Here's how the part is built. I have some questions about the finished solid (model axes, mm). A direction names the side the tool comes from. Coordinates: 2 decimals unless noted, no trailing zeros. Loops run counter-clockwise (first coordinate to the right, second up) from the corner with the lowest first, then second, coordinate; pieces in that order, holes last. Notation, with made-up numbers: (-35, -5) -> (-18, -5) arc R32 cw to (-18, 33) -> close; hole circle Ø1 at (4.5, 63). An arc over 180 degrees is marked (long way). Answer as a JSON object with one key per item and string values. Group by question number.
Q1. I want a section at B-B on z = 2.2. Write out the boundary of the cut face in (x, y).
Q2. On a 3-axis mill with a long thin cutter (end or side, diameter ignored), from which of +Z, -Z, +X, -X, +Y, -Y can I reach the whole of each face in a straight line? I mean faces 1 (the flat face through (5, 4, 0.6)), 2 (the flat face through (5, -10, 5)). Say none if no direction works.
Q3. I want a section at A-A on x = 5. Write out the boundary of the cut face in (y, z).
Q4. I need wall thicknesses on line 1 (Z direction, x = 8, y = 5); line 2 (Y direction, x = 4.25, z = 3); line 3 (Y direction, x = 5, z = 2.25). Which ranges of each line are inside material? Lowest first, please.
Q5. I'm going to push flat-ended pins straight in: pin 1 (2 mm diameter, centred on x = 8, z = 4, fed in from +Y); pin 2 (3 mm diameter, centred on x = 3, z = 3, fed in from +Y). Where does each tip first touch, or does it pass through?
Q6. I want a section at C-C on y = -0.75. Write out the boundary of the cut face in (x, z).
```python
from build123d import *

# Parameters (mm, degrees)
F0_W        = 10
F0_H        = 10
F0_H_2      = 2
F0_H_3      = 12
F1_DEPTH    = 0.6
F2_DEPTH    = 5
F3_T4_DEPTH = 35.7168298797


# Not quite as in the source:
# - a fillet or chamfer that OpenCascade refuses, or shapes differently, is made with other operations: its cross-section is extruded or revolved along the edge and cut away or added


with BuildPart() as f1:
    # F0 (on Top) → F1 (new body)
    with BuildSketch(Plane.XY):
        with Locations((5, 5)):
            Rectangle(F0_W, F0_H)
        with Locations((5, -1)):
            Rectangle(F0_W, F0_H_2)
        with Locations((5, -8)):
            Rectangle(F0_W, F0_H_3)
    extrude(amount=F1_DEPTH)

    # F0 (on Top) → F2 (join)
    with BuildSketch(Plane.XY):
        with Locations((5, -8)):
            Rectangle(F0_W, F0_H_3)
    extrude(amount=F2_DEPTH)

    # F3: chamfer of 5 on 1 edges, made by hand


with BuildPart() as f3_tool2:
    # F3_s3 → F3_t4 (new body)
    with BuildSketch(Plane.YZ.offset(22.8584149398)):
        Polygon((-7, 5), (-2, 0), (-2, 5), align=None)
    extrude(amount=-F3_T4_DEPTH)

    split(bisect_by=Plane.XY.offset(0.6), keep=Keep.TOP)


with BuildPart() as f1_1:
    add(f1.part)

    # F3_t1: cut F3_tool2
    add(f3_tool2.part, mode=Mode.SUBTRACT)


solid = f1_1.part
```
Result set:
{
 "1": {"outline": "(0, -14) -> (10, -14) -> (10, -4.2) -> (0, -4.2) -> close"},
 "2": {"face 1": "+Z, +X, -X, +Y", "face 2": "+Z, +X, -X, +Y, -Y"},
 "3": {"outline": "(-14, 0) -> (10, 0) -> (10, 0.6) -> (-2.6, 0.6) -> (-7, 5) -> (-14, 5) -> close"},
 "4": {"line 1": "z = 0 to 0.6", "line 2": "y = -14 to -5", "line 3": "y = -14 to -4.25"},
 "5": {"pin 1": "stops at y = -5", "pin 2": "stops at y = -3.5"},
 "6": {"outline": "(0, 0) -> (10, 0) -> (10, 0.6) -> (0, 0.6) -> close"}
}
